Part model, mm, in its own coordinate system. Face numbers are marked on the shaded views. A direction names the side the tool comes from. Give positions to 0.01 mm unless a question says otherwise; leave off trailing zeros. Order: outer loops, then holes, each group sorted by start corner. A loop starts at its lowest first (then second) coordinate and runs counter-clockwise, first axis right, second up. Notation, with made-up numbers: M 66,78 L 110,78 A28 ccw 110,106 Z; hole C 50.5,-38 d5. An arc over 180 degrees is marked long. Answer as a JSON object with one key per item and string values.
Autodesk Inventor part; units mm, degrees
ref_plane "YZ Plane" through (0, 0, 0) normal (1, 0, 0) x (0, 1, 0)
ref_plane "XZ Plane" through (0, 0, 0) normal (0, 1, 0) x (-1, 0, 0)
ref_plane "XY Plane" through (0, 0, 0) normal (0, 0, 1) x (1, 0, 0)
sketch "Sketch2" plane through (0, 0, 0) normal (0, 1, 0) x (-1, 0, 0)
  line L0 (0, 0) -> (-48, 0)
  line L1 (-48, 0) -> (-48, -79.835)
  line L2 (-48, -79.835) -> (0, -79.835)
  line L3 (-40, -59.9175) -> (-9, -59.9175)
  line L4 (-9, -59.9175) -> (-9, -19.9175)
  line L5 (-9, -19.9175) -> (-40, -19.9175)
  line L6 (-33.9858, -17.4175) -> (3.086, -17.4175)
  line L7 (3.086, -62.4175) -> (-40, -62.4175)
  line L8 (-48, -6) -> (-48, -3.5)
  line L9 (-33.9858, -17.4175) -> (-40, -17.4175)
  line L10 (-40, -62.4175) -> (-40, -59.9175)
  line L11 (-40, -19.9175) -> (-40, -17.4175)
  line L12 (3.086, -16.9175) -> (-40.5, -16.9175)
  line L13 (-40.5, -16.9175) -> (-40.5, -20.4175)
  line L14 (-40.5, -20.4175) -> (-9.5, -20.4175)
  line L15 (-9.5, -20.4175) -> (-9.5, -59.4175)
  line L16 (-9.5, -59.4175) -> (-40.5, -59.4175)
  line L17 (-40.5, -59.4175) -> (-40.5, -62.9175)
  line L18 (-40.5, -62.9175) -> (3.086, -62.9175)
  line L19 (5, -12.8942) -> (5, -16.38)
  line L20 (0, 0) -> (3.086, 0)
  line L21 (3.086, 0) -> (3.086, -79.835)
  line L22 (3.086, -79.835) -> (0, -79.835)
  line L23 (3.086, -62.9175) -> (3.086, -62.4175)
  line L24 (3.086, -17.4175) -> (3.086, -16.9175)
  line L25 (3.086, -62.9175) -> (3.086, -62.4175)
  line L26 (3.086, -17.4175) -> (3.086, -16.9175)
  line L27 (-9.5, -27.9375) -> (-40.5, -27.9375)
  line L28 (-40.5, -27.9375) -> (-40.5, -51.8975)
  line L29 (-40.5, -51.8975) -> (-9.5, -51.8975)
  line L30 (-9.5, -51.8975) -> (-9.5, -27.9375)
  point P0 (-9.7436, -6)
  point P1 (0, -79.835)
  point P2 (-9.5, -51.8975)
  dimension "d19" = 79.835
  dimension "d20" = 45
  dimension "d21" = 17.4175
  dimension "d22" = 2.5
  dimension "d23" = 40
  dimension "d24" = 39
  dimension "d26" = 0.5
  dimension "d32" = 7.52
  dimension "d33" = 7.52
  dimension "d34" = 23.96
  dimension "d35" = 51.086
extrude "Extrusion7" add sketch "Sketch2" along normal blind 60 contours L20 L21 L12 L13 L14 L15 L27 L28 L29 L16 L17 L18 L22 L2 L1 L0
sketch "Sketch3" plane through (-3.086, 0, 0) normal (0, 0, 1) x (1, 0, 0)
  circle A0 centre (22.5, 51.8947) radius 2.8
  circle A1 centre (22.5, 19.8947) radius 2.8
  point P0 (3.086, 0)
  dimension "d38" = 32
extrude "Extrusion8" cut sketch "Sketch3" against normal through all
sketch "Sketch4" plane through (-3.086, 0, -79.835) normal (-1, 0, 0) x (0, 0, 1)
  circle A0 centre (7.9375, 41) radius 2.5
  circle A1 centre (7.9375, 9) radius 2.5
  line L0 (0, 0) -> (16.9175, 0)
  circle A2 centre (55.9175, 52.5) radius 1.5
  circle A3 centre (23.9175, 52.5) radius 1.5
  point P0 (79.835, 0)
  dimension "d36" = 5
  dimension "d37" = 5
  dimension "d39" = 32
  dimension "d40" = 9
  dimension "d43" = 3
extrude "Extrusion9" cut sketch "Sketch4" against normal blind 20 contours A0 | A1
extrude "Extrusion10" cut sketch "Sketch4" along normal blind 10 from surface at -51.086 contours A2 | A3
equation "\"d21\" = -0.5 * d20 + 0.5 * d19"
equation "\"d33\" = d32"
properties part number "Intake Mounting Block"
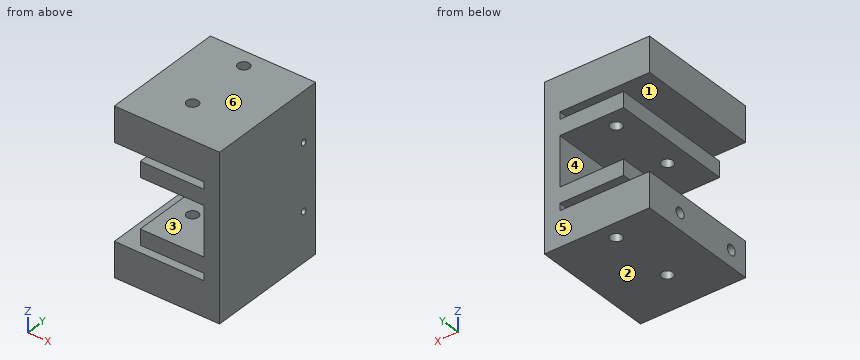
1. Which spindle directions (+Z, -Z, +X, -X, +Y, -Y) get a long thin tool onto all of the face, cutting with end or side? Do the marked faces 1 and 2. Say none if no direction does.
Worked answers:
{"face 1": "-X, +Y, -Y", "face 2": "-Z, +X, -X, +Y, -Y"}
2. Cut at C-C on y = 41. Give the cut face in (x, z) (1 decimal), plus the area to 3 significant figures.
Worked answers:
{"outline": "M -3.1,-79.8 L 48,-79.8 L 48,0 L -3.1,0 L -3.1,-16.9 L 40.5,-16.9 L 40.5,-20.4 L 9.5,-20.4 L 9.5,-27.9 L 40.5,-27.9 L 40.5,-51.9 L 9.5,-51.9 L 9.5,-59.4 L 40.5,-59.4 L 40.5,-62.9 L -3.1,-62.9 L -3.1,-69.4 L 16.9,-69.4 L 16.9,-74.4 L -3.1,-74.4 Z", "area": "2,440 mm^2"}
3. Cut at A-A on x = 15. Give the cut face in (y, z) (1 decimal), plus the area to 3 significant figures.
Worked answers:
{"outline": "M 0,-79.8 L 60,-79.8 L 60,-62.9 L 0,-62.9 Z; M 0,-59.4 L 60,-59.4 L 60,-51.9 L 0,-51.9 Z; M 0,-27.9 L 60,-27.9 L 60,-20.4 L 0,-20.4 Z; M 0,-16.9 L 60,-16.9 L 60,0 L 0,0 Z; hole C 9,-71.9 d5; hole C 41,-71.9 d5", "area": "2,890 mm^2"}
4. Cut at D-D on z = -68.5. Give the cut face in (x, y).
Worked answers:
{"outline": "M -3.09,0 L 48,0 L 48,60 L -3.09,60 Z; hole C 19.41,19.89 d5.6; hole C 19.41,51.89 d5.6"}
5. Pin check, flat tip, straight feed: P1, Ø4.5, axis at y = 9, z = -71.9, coming from the -X side. Stop position of the tip, or through.
Worked answers:
{"P1": "stops at x = 16.91"}
6. Probe line 1 along Z through (x, y) = (13, 21.5) (1 decimal); line 2 along X through (y, z) = (52, -64.5); line 3 along Y through (x, z) = (20.5, -52). List the from-to ranges inside material, lowest first.
Worked answers:
{"line 1": "z = -79.8 to -62.9, -59.4 to -51.9, -27.9 to -20.4, -16.9 to 0", "line 2": "x = -3.09 to 16.62, 22.21 to 48", "line 3": "y = 0 to 17.31, 22.48 to 49.31, 54.48 to 60"}
7. Cut at B-B on x = 28.5. Give the cut face in (y, z) (1 decimal), plus the area to 3 significant figures.
Worked answers:
{"outline": "M 0,-79.8 L 60,-79.8 L 60,-62.9 L 0,-62.9 Z; M 0,-59.4 L 60,-59.4 L 60,-51.9 L 0,-51.9 Z; M 0,-27.9 L 60,-27.9 L 60,-20.4 L 0,-20.4 Z; M 0,-16.9 L 60,-16.9 L 60,0 L 0,0 Z", "area": "2,930 mm^2"}
8. Two-plate mould, pull along Z, no slides. Class the marked faces 3, 4, 5 and 6: +Z half, -Z half, draft (parallel to the pull), parting line (faces both ways), or undercut.
Worked answers:
{"face 3": "undercut", "face 4": "undercut", "face 5": "draft", "face 6": "+Z half"}
